```python
from build123d import *

# Parameters (mm, degrees)
BOSS_EXTRUDE1_DEPTH = 3


with BuildPart() as part:
    # Sketch1 → Boss-Extrude1 (new body)
    with BuildSketch(Plane(origin=(0, 0, 0), x_dir=(0, 0, -1), z_dir=(1, 0, 0))):
        with BuildLine():
            Line((24.704010852, 12.720489708), (33.704010852, 12.720489708))
            ThreePointArc((33.704010852, 12.720489708), (38.387131684, 10.663164706), (39.704010852, 5.720489708))
            Line((39.704010852, 5.720489708), (39.704010852, -1.279510292))
            Line((39.704010852, -1.279510292), (46.704010852, -1.279510292))
            Line((46.704010852, -1.279510292), (46.704010852, 8.720489708))
            Line((46.704010852, 8.720489708), (49.704010852, 8.720489708))
            Line((49.704010852, 8.720489708), (49.704010852, 18.720489708))
            Line((49.704010852, 18.720489708), (46.704010852, 18.720489708))
            Line((46.704010852, 18.720489708), (46.704010852, 28.720489708))
            Line((46.704010852, 28.720489708), (49.704010852, 28.720489708))
            Line((49.704010852, 28.720489708), (49.704010852, 38.720489708))
            Line((49.704010852, 38.720489708), (46.704010852, 38.720489708))
            Line((46.704010852, 38.720489708), (46.704010852, 48.720489708))
            Line((46.704010852, 48.720489708), (49.704010852, 48.720489708))
            Line((49.704010852, 48.720489708), (49.704010852, 58.720489708))
            Line((49.704010852, 58.720489708), (46.704010852, 58.720489708))
            Line((46.704010852, 58.720489708), (46.704010852, 68.720489708))
            Line((46.704010852, 68.720489708), (49.704010852, 68.720489708))
            Line((49.704010852, 68.720489708), (49.704010852, 78.720489708))
            Line((49.704010852, 78.720489708), (46.704010852, 78.720489708))
            Line((46.704010852, 78.720489708), (46.704010852, 88.720489708))
            Line((46.704010852, 88.720489708), (39.704010852, 88.720489708))
            Line((39.704010852, 88.720489708), (39.704010852, 85.720489708))
            Line((39.704010852, 85.720489708), (29.704010852, 85.720489708))
            Line((29.704010852, 85.720489708), (29.704010852, 88.720489708))
            Line((29.704010852, 88.720489708), (24.704010852, 88.720489708))
            Line((24.704010852, 88.720489708), (24.704010852, 12.720489708))
        make_face()
    extrude(amount=BOSS_EXTRUDE1_DEPTH)


solid = part.part
```
Geometry: final body of the model. Coordinates: model frame, mm. A direction names the side the tool comes from. Round coordinates to 2 decimals unless told otherwise and drop trailing zeros. Loops run counter-clockwise (first coordinate to the right, second up) from the corner with the lowest first, then second, coordinate; pieces in that order, holes last. Notation, with made-up numbers: (78, -13.75) -> (93, -13.75) arc R5 ccw to (93, -9.75) -> close; hole circle Ø11 at (77.25, 44). An arc over 180 degrees is marked (long way). Use one line per item in the form item = value. Start each with the question number.
1) Line query: L1, parallel to Y at x = 0.5, z = -47; L2, parallel to Z at x = 2.55, y = 48; L3, parallel to Y at x = 0.95, z = -32.5. Output: solid intervals per line, ascending.
2) First-contact query: P1, Ø1.5, axis at x = 2, z = -48.5, coming from the -Y side; P2, Ø0.9, axis at x = 2, y = 44, coming from the -Z side; P3, Ø1.5, axis at x = 1.5, z = -34, coming from the +Y side. Flat tips, straight axial feed; report the tip coordinate or a pass-through.
3) Draft query along Z for faces 5 (the flat face through (1, 44, -46.704)), 6 (the flat face through (1, 87, -29.704)), 7 (the flat face through (1, 18.72, -48)). Return one class per face: released by +Z, released by -Z, zero draft, split by the parting line, or undercut.
4) Section A-A on x = 1.35. Output: boundary loops of the cut face in (y, z).
5) Section B-B on y = 59.5. Output: boundary loops of the cut face in (x, z), then the cut area to 3 significant figures.
6) Section C-C on z = -26.5. Output: boundary loops of the cut face in (x, y).
7) Access query for faces 1 (the flat face through (1, 78.72, -48)), 2 (the flat face through (1, 12.72, -29)), 3 (the flat face through (1, 85.72, -35)), 4 (the flat face through (1, 28.72, -48)). Directions: +Z, -Z, +X, -X, +Y, -Y. A direction counts if a zero-diameter tool reaches every point of the face in a straight line with its end or side. Return the directions, or none.
Response:
q1.L1 = 8.72 to 18.72, 28.72 to 38.72, 48.72 to 58.72, 68.72 to 78.72
q1.L2 = -46.7 to -24.7
q1.L3 = 12.72 to 85.72
q2.P1 = 8.72
q2.P2 = -46.7
q2.P3 = 85.72
q3.face_5 = released by -Z
q3.face_6 = undercut
q3.face_7 = zero draft
q4.outline = (-1.28, -46.7) -> (8.72, -46.7) -> (8.72, -49.7) -> (18.72, -49.7) -> (18.72, -46.7) -> (28.72, -46.7) -> (28.72, -49.7) -> (38.72, -49.7) -> (38.72, -46.7) -> (48.72, -46.7) -> (48.72, -49.7) -> (58.72, -49.7) -> (58.72, -46.7) -> (68.72, -46.7) -> (68.72, -49.7) -> (78.72, -49.7) -> (78.72, -46.7) -> (88.72, -46.7) -> (88.72, -39.7) -> (85.72, -39.7) -> (85.72, -29.7) -> (88.72, -29.7) -> (88.72, -24.7) -> (12.72, -24.7) -> (12.72, -33.7) arc R5.9 cw to (5.72, -39.7) -> (-1.28, -39.7) -> close
q5.outline = (0, -46.7) -> (3, -46.7) -> (3, -24.7) -> (0, -24.7) -> close
q5.area = 66.0 mm^2
q6.outline = (0, 12.72) -> (3, 12.72) -> (3, 88.72) -> (0, 88.72) -> close
q7.face_1 = -Z, +X, -X, +Y
q7.face_2 = +Z, +X, -X, -Y
q7.face_3 = +X, -X, +Y
q7.face_4 = -Z, +X, -X
